Check sheet for the modelled part. Datum: model origin and axes. Units: mm. Round coordinates to 2 decimals unless told otherwise and drop trailing zeros. Loops run counter-clockwise (first coordinate to the right, second up) from the corner with the lowest first, then second, coordinate; pieces in that order, holes last. Notation, with made-up numbers: (-24.5, 51.25) -> (15.5, 51.25) arc R19 ccw to (15.5, 69.25) -> close; hole circle Ø2 at (65.25, -16). An arc over 180 degrees is marked (long way). Return JSON: item names as keys, results as strings.
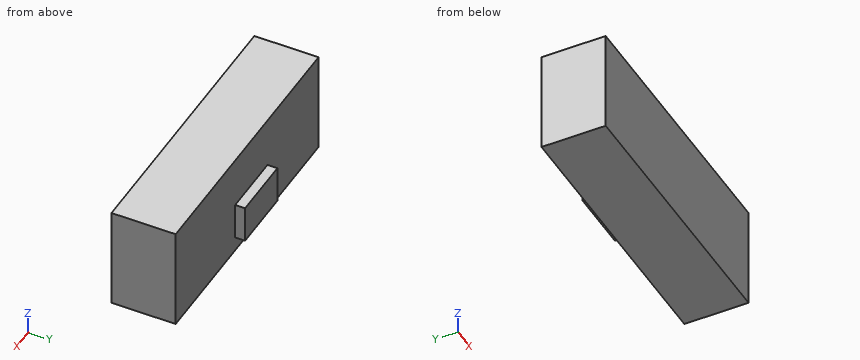
from build123d import *

# Parameters (mm, degrees)
SK_P01_F2INLINEHOLDER5A_W        = 56
SK_P01_F2INLINEHOLDER5A_H        = 21
P01_F2INLINEHOLDER5A_DEPTH       = 13
P02_D1IDEALDIODEPOLOLU5382_START = 13
SK_P02_D1IDEALDIODEPOLOLU5382_W  = 12.7
SK_P02_D1IDEALDIODEPOLOLU5382_H  = 7.6
P02_D1IDEALDIODEPOLOLU5382_DEPTH = 2


with BuildPart() as part:
    # SK_P01_F2inlineholder5A → P01_F2inlineholder5A (new body)
    with BuildSketch(Plane(origin=(0, 0, 0), x_dir=(1, 0, 0), z_dir=(0, 1, 0))):
        Rectangle(SK_P01_F2INLINEHOLDER5A_W, SK_P01_F2INLINEHOLDER5A_H)
    extrude(amount=P01_F2INLINEHOLDER5A_DEPTH)

    # SK_P02_D1idealdiodePololu5382 → P02_D1idealdiodePololu5382 (add)
    with BuildSketch(Plane(origin=(0, 0, 0), x_dir=(1, 0, 0), z_dir=(0, 1, 0)).offset(P02_D1IDEALDIODEPOLOLU5382_START)):
        with Locations((-1.65, 3.7)):
            Rectangle(SK_P02_D1IDEALDIODEPOLOLU5382_W, SK_P02_D1IDEALDIODEPOLOLU5382_H)
    extrude(amount=P02_D1IDEALDIODEPOLOLU5382_DEPTH)


solid = part.part
Q1. Section check C-C (x = 12.5). Record the boundary of the cut face in (y, z).
Results list:
{"outline": "(0, -10.5) -> (13, -10.5) -> (13, 10.5) -> (0, 10.5) -> close"}
Q2. Go/stop test with flat-tipped pins: pin 1 (10 mm diameter, centred on x = -13.5, z = 7.5, fed in from +Y); pin 2 (1.6 mm diameter, centred on y = 14, z = -5.5, fed in from -X); pin 3 (1 mm diameter, centred on x = 0, y = 14.5, fed in from +Z). Record where each tip stops, or that it passes through.
Results list:
{"pin 1": "y = 13", "pin 2": "x = -8", "pin 3": "z = 0.1"}
Q3. Material ranges on line 1 (Y direction, x = -3.5, z = 3); line 2 (Z direction, x = -3, y = 14); line 3 (X direction, y = 13.25, z = -1.75), recorded low to high.
Results list:
{"line 1": "0 to 13", "line 2": "-7.5 to 0.1", "line 3": "-8 to 4.7"}
Q4. Section check A-A (z = -1). Record the boundary of the cut face in (x, y).
Results list:
{"outline": "(-28, 0) -> (28, 0) -> (28, 13) -> (4.7, 13) -> (4.7, 15) -> (-8, 15) -> (-8, 13) -> (-28, 13) -> close"}
Q5. Section check B-B (y = 13.75). Record the boundary of the cut face in (x, z), then the cut area to 3 significant figures.
Results list:
{"outline": "(-8, -7.5) -> (4.7, -7.5) -> (4.7, 0.1) -> (-8, 0.1) -> close", "area": "96.5 mm^2"}
